For this review, take the finished solid that the model builds, in its own axes (mm). Face numbers are marked on the shaded views. A direction names the side the tool comes from. Give positions to 0.01 mm unless a question says otherwise; leave off trailing zeros. Loops run counter-clockwise (first coordinate to the right, second up) from the corner with the lowest first, then second, coordinate; pieces in that order, holes last.
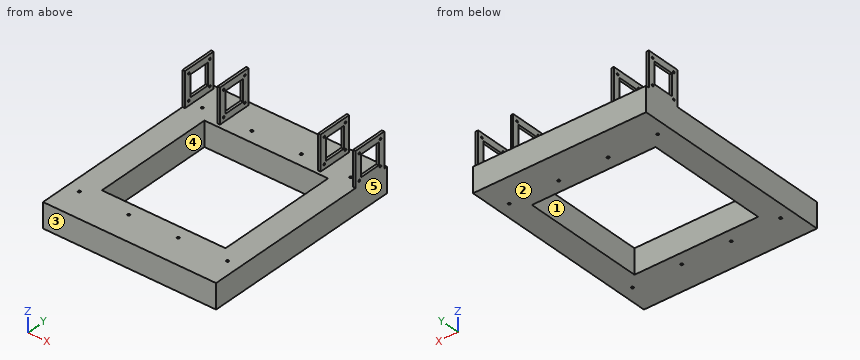
Autodesk Inventor part; units mm, degrees
ref_plane "XZ Plane" through (0, 0, 0) normal (0, 1, 0) x (-1, 0, 0)
ref_plane "XY Plane" through (0, 0, 0) normal (0, 0, 1) x (1, 0, 0)
sketch "Эскиз1" plane through (0, 0, 0) normal (0, 0, 1) x (1, 0, 0)
  line L0 (75, -75) -> (-75, -75)
  line L1 (-75, -75) -> (-75, 75)
  line L2 (-75, 75) -> (75, 75)
  line L3 (75, 75) -> (75, -75)
  line L4 (105, -125) -> (-105, -125)
  line L5 (-105, -125) -> (-105, 125)
  line L6 (-105, 125) -> (105, 125)
  line L7 (105, 125) -> (105, -125)
  point P0 (0, 0)
  point P1 (-75, 0)
  point P2 (0, -125)
  point P3 (-105, 0)
  dimension "d0" = 210
  dimension "d1" = 250
  dimension "d3" = 150
  dimension "d4" = 150
  dimension "d5" = 125
  dimension "d6" = 105
  dimension "d7" = 75
  dimension "d8" = 75
extrude "Выдавливание1" add sketch "Эскиз1" along normal blind 30
sketch "Эскиз2" plane through (0, 0, 30) normal (0, 0, 1) x (1, 0, 0)
  circle A0 centre (90, -90) radius 1.5
  line L0 (75, 75) -> (75, -75)
  line L1 (-105, 125) -> (-105, -125)
  line L2 (90, -90) -> (84.6408, -90) construction
  line L3 (84.6408, -90) -> (90, -90)
  line L4 (90, -90) -> (90, -87.0291) construction
  circle A1 centre (-90, -90) radius 1.5
  circle A2 centre (90, 90) radius 1.5
  circle A3 centre (-90, 90) radius 1.5
  circle A4 centre (30, 90) radius 1.5
  circle A5 centre (30, -90) radius 1.5
  circle A6 centre (-30, 90) radius 1.5
  circle A7 centre (-30, -90) radius 1.5
  point P0 (0, 0)
  point P1 (75, 0)
  dimension "d11" = 3
  dimension "d12" = 90
  dimension "d13" = 195
  dimension "d16" = 180
  dimension "d19" = 180
  dimension "d24" = 60
extrude "Выдавливание2" cut sketch "Эскиз2" against normal through all
ref_plane "РабПлоскость4" through (19.7, 0, 0) normal (1, 0, 0) x (0, 1, 0)
sketch "Эскиз7" plane through (105, 0, 0) normal (1, 0, 0) x (0, 1, 0)
  line L0 (79, 30) -> (121, 30)
  line L1 (121, 30) -> (121, 38)
  line L2 (121, 38) -> (79, 38)
  line L3 (79, 38) -> (79, 30)
  line L4 (121, 30) -> (113, 30)
  line L5 (113, 30) -> (113, 72)
  line L6 (113, 72) -> (121, 72)
  line L7 (121, 72) -> (121, 30)
  line L8 (121, 72) -> (79, 72)
  line L9 (79, 72) -> (79, 64)
  line L10 (79, 64) -> (121, 64)
  line L11 (121, 64) -> (121, 72)
  line L12 (79, 72) -> (87, 72)
  line L13 (87, 72) -> (87, 30)
  line L14 (87, 30) -> (79, 30)
  line L15 (79, 30) -> (79, 72)
  line L16 (75, 30) -> (125, 30) construction
  circle A0 centre (84.5, 66.5) radius 1.25
  circle A1 centre (115.5, 66.5) radius 1.25
  circle A2 centre (115.5, 35.5) radius 1.25
  circle A3 centre (84.5, 35.5) radius 1.25
  point P0 (0, 0)
  point P1 (117, 72)
  point P2 (113, 38)
  point P3 (87, 38)
  point P4 (87, 64)
  point P5 (113, 64)
  dimension "d80" = 42
  dimension "d81" = 42
  dimension "d82" = 8
  dimension "d83" = 8
  dimension "d84" = 4
  dimension "d85" = 8
  dimension "d86" = 8
  dimension "d87" = 2.5
  dimension "d88" = 5.5
  dimension "d89" = 5.5
  dimension "d90" = 2.5
  dimension "d91" = 2.5
  dimension "d92" = 2.5
  dimension "d93" = 5.5
  dimension "d94" = 5.5
  dimension "d95" = 5.5
  dimension "d96" = 5.5
  dimension "d97" = 5.5
  dimension "d98" = 5.5
extrude "Выдавливание5" add sketch "Эскиз7" against normal blind 3 contours L3 L2 L13 L0 | L13 L2 L5 L0 | L15 L10 L13 L2 | L5 L2 L1 L0 | L9 L8 L13 L10 | L5 L10 L7 L2 | L13 L8 L5 L10 | L5 L6 L7 L10
mirror "Зеркальное отражение3" about plane through (0, 0, 0) normal (1, 0, 0) of "Выдавливание5"
ref_plane "РабПлоскость5" through (62.5, -125, 0) normal (1, 0, 0) x (0, 0, -1)
sketch "Эскиз8" plane through (62.5, -125, 0) normal (1, 0, 0) x (0, 0, -1)
  line L0 (-30, 204) -> (-30, 250) construction
  line L1 (-30, 204) -> (-38, 204)
  line L2 (-38, 204) -> (-38, 246)
  line L3 (-38, 246) -> (-30, 246)
  line L4 (-30, 246) -> (-30, 204)
  line L5 (-30, 246) -> (-72, 246)
  line L6 (-72, 246) -> (-72, 238)
  line L7 (-72, 238) -> (-30, 238)
  line L8 (-30, 238) -> (-30, 246)
  line L9 (-72, 246) -> (-64, 246)
  line L10 (-64, 246) -> (-64, 204)
  line L11 (-64, 204) -> (-72, 204)
  line L12 (-72, 204) -> (-72, 246)
  line L13 (-72, 204) -> (-30, 204)
  line L14 (-30, 204) -> (-30, 212)
  line L15 (-30, 212) -> (-72, 212)
  line L16 (-72, 212) -> (-72, 204)
  circle A0 centre (-66.5, 209.5) radius 1.25
  circle A1 centre (-66.5, 240.5) radius 1.25
  circle A2 centre (-35.5, 240.5) radius 1.25
  circle A3 centre (-35.5, 209.5) radius 1.25
  point P0 (0, 125)
  point P1 (-34, 204)
  point P2 (-30, 242)
  point P3 (-38, 238)
  point P4 (-38, 212)
  point P5 (-64, 212)
  point P6 (-64, 238)
  dimension "d102" = 8
  dimension "d103" = 8
  dimension "d104" = 8
  dimension "d105" = 8
  dimension "d106" = 42
  dimension "d107" = 4
  dimension "d108" = 42
  dimension "d109" = 5.5
  dimension "d110" = 5.5
  dimension "d111" = 5.5
  dimension "d112" = 5.5
  dimension "d113" = 5.5
  dimension "d114" = 5.5
  dimension "d115" = 5.5
  dimension "d116" = 5.5
  dimension "d117" = 2.5
  dimension "d118" = 2.5
  dimension "d119" = 2.5
  dimension "d120" = 2.5
extrude "Выдавливание6" add sketch "Эскиз8" against normal blind 3 contours L1 L2 L15 L4 | L13 L10 L15 L2 | L15 L2 L7 L4 | L11 L12 L15 L10 | L7 L2 L3 L4 | L7 L10 L5 L2 | L15 L12 L7 L10 | L7 L6 L5 L10
mirror "Зеркальное отражение4" about plane through (0, 0, 0) normal (1, 0, 0) of "Выдавливание6"
properties part number "ОСНОВА"
Item 1: Clearance check with flat-ended pins moving along their axes: pin 1 Ø12.5 at (y, z) = (98.5, 53.5) entering from +X; pin 2 Ø2.5 at (x, z) = (61.5, 52.5) entering from -Y; pin 3 Ø3 at (y, z) = (84.5, 35.5) entering from +X; pin 4 Ø0.9 at (x, z) = (-103, 60) entering from +Y. State where each tip first meets the part, or that it passes through.
Answer:
pin 1: passes through
pin 2: stops at y = 79
pin 3: stops at x = 105
pin 4: stops at y = 121
Item 2: Take a section at C-C on x = 18.5. Give the boundary of the cut face in (y, z), and give its area (3 significant figures).
Answer:
outline: (-125, 0) - (-75, 0) - (-75, 30) - (-125, 30) - close; (75, 0) - (125, 0) - (125, 30) - (75, 30) - close
area: 3,000 mm2
Item 3: For L1, parallel to X at y = 103.5, z = 34.5; L2, parallel to X at y = -90, z = 6; L3, parallel to Y at x = 61.15, z = 66.5, list the stretches that pass through material, from the lowest coordinate up.
Answer:
L1: x = -105 to -102, -62.5 to -59.5, 59.5 to 62.5, 102 to 105
L2: x = -105 to -91.5, -88.5 to -31.5, -28.5 to 28.5, 31.5 to 88.5, 91.5 to 105
L3: y = 79 to 83.25, 85.75 to 114.25, 116.75 to 121
Item 4: Take a section at B-B on z = 51. State how many separate pieces and enclosed holes the cut face has, and give its area (3 significant figures).
Answer:
separate pieces: 8
enclosed holes: 0
area: 192 mm2
Item 5: Take a section at A-A on y = 38. Give the boundary of the cut face in (x, z), and give its area (3 significant figures).
Answer:
outline: (-105, 0) - (-75, 0) - (-75, 30) - (-105, 30) - close; (75, 0) - (105, 0) - (105, 30) - (75, 30) - close
area: 1,800 mm2
Item 6: Tool access review of the marked faces 1 and 2: name each direction out of +Z, -Z, +X, -X, +Y, -Y from which nothing blocks a thin tool from reaching the whole face with its end or side.
Answer:
face 1: +Z, -Z
face 2: -Z, +X, -X, +Y, -Y
Item 7: The part is to be moulded in two halves that separate along X. For the marked faces 3, 4 and 5, say which applies: released by +X, released by -X, zero draft, split by the parting line, or undercut.
Answer:
face 3: zero draft
face 4: undercut
face 5: released by +X
